Source: CAD feature listing. Evaluate the final solid. Frame: model axes, mm. Face numbers are marked on the shaded views. Coordinates: 2 decimals unless noted, no trailing zeros. Write each loop counter-clockwise with the first axis right and the second up, starting at its lowest first coordinate (ties: lowest second). Pieces come first, ordered by that corner, then holes. Notation, with made-up numbers: (76.25, 18) - (106.25, 18) arc R29 ccw to (106.25, 41) - close; hole circle Ø11 at (8.5, -24). An arc over 180 degrees is marked (long way). One line per question, with ' | ' between items. Start each with the question number.
Q1. Cut plane A-A, the plane z = -6.75. Return loops of the section in (x, y), plus the area to 3 significant figures.
Q2. Line query: line 1 (Y direction, x = 1.6, z = -5); line 2 (Z direction, x = 0.55, y = -9); line 3 (Y direction, x = 1, z = -3.25). Output: solid intervals per line, ascending.
Q3. Cut plane D-D, the plane z = -8.75. Return loops of the section in (x, y).
Q4. Cut plane C-C, the plane x = 0.85. Return loops of the section in (y, z), plus the area to 3 significant figures.
Q5. Draft query along Z for the marked faces 1, 2, 3 and 4. Return one class per face: +Z half, -Z half, draft (parallel to the pull), parting line (faces both ways), or undercut.
Q6. Cut plane B-B, the plane y = -9. Return loops of the section in (x, z), plus the area to 3 significant figures.
Autodesk Inventor part; units mm, degrees
ref_plane "YZ Plane" through (0, 0, 0) normal (1, 0, 0) x (0, 1, 0)
ref_plane "XZ Plane" through (0, 0, 0) normal (0, 1, 0) x (-1, 0, 0)
ref_plane "XY Plane" through (0, 0, 0) normal (0, 0, 1) x (1, 0, 0)
sketch "Esboço1" plane through (0, 0, 0) normal (1, 0, 0) x (0, 1, 0)
  line L0 (0, 0) -> (-11, 0)
  line L1 (-15, -4) -> (-15, -6)
  line L2 (-11, -10) -> (0, -10)
  line L3 (0, -10) -> (0, 0)
  arc A0 (-11, 0) -> (-15, -4) centre (-11, -4) ccw
  arc A1 (-15, -6) -> (-11, -10) centre (-11, -6) ccw
  line L4 (-15, -5) -> (-9, -5)
  circle A2 centre (-9, -5) radius 3
  point P0 (-15, -10)
  point P1 (-15, 0)
  dimension "d0" = 15
  dimension "d1" = 10
  dimension "d2" = 4
  dimension "d3" = 6
  dimension "d4" = 6
extrude "Extrusão1" add sketch "Esboço1" along normal blind 2
sketch "Esboço2" plane through (2, 0, 0) normal (1, 0, 0) x (0, 0, -1)
  circle A0 centre (5, -9) radius 3
properties part number "Chapa da Luz de Freio"
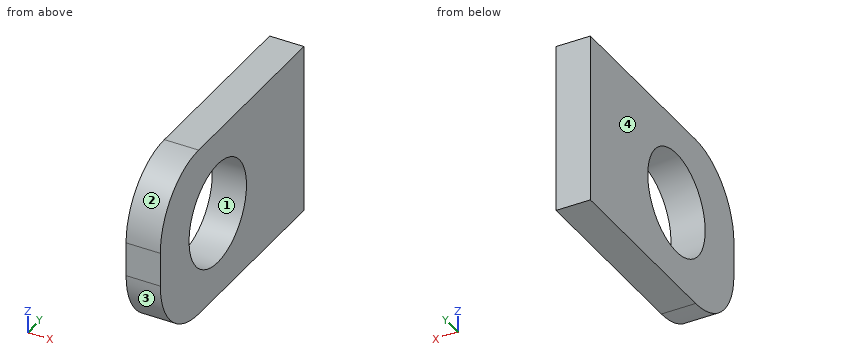
Reply:
1) outline: (0, -14.93) - (2, -14.93) - (2, -11.44) - (0, -11.44) - close; (0, -6.56) - (2, -6.56) - (2, 0) - (0, 0) - close | area: 20.1 mm^2
2) line 1: y = -15 to -12, -6 to 0 | line 2: z = -10 to -8, -2 to 0 | line 3: y = -14.93 to -11.44, -6.56 to 0
3) outline: (0, -13.9) - (2, -13.9) - (2, 0) - (0, 0) - close
4) outline: (-15, -6) arc R4 ccw to (-11, -10) - (0, -10) - (0, 0) - (-11, 0) arc R4 ccw to (-15, -4) - close; hole circle Ø6 at (-9, -5) | area: 115 mm^2
5) face 1: undercut | face 2: +Z half | face 3: -Z half | face 4: draft
6) outline: (0, -10) - (2, -10) - (2, -8) - (0, -8) - close; (0, -2) - (2, -2) - (2, 0) - (0, 0) - close | area: 8.00 mm^2
